from build123d import *

# Parameters (mm, degrees)
F0_R     = 40.75
F0_R_2   = 39.55
F1_DEPTH = 50
F0_R_3   = 57.8499995172
F0_R_4   = 43.75
F0_R_5   = 42.55
F2_DEPTH = 1
F3_DEPTH = 50


with BuildPart() as f1:
    # F0 (on Top) → F1 (new body)
    with BuildSketch(Plane.XY):
        Circle(F0_R)
        Circle(F0_R_2, mode=Mode.SUBTRACT)
    extrude(amount=-F1_DEPTH)

    # F0 (on Top) → F2 (join)
    with BuildSketch(Plane.XY):
        Circle(F0_R_3)
        Circle(F0_R_4, mode=Mode.SUBTRACT)
        Circle(F0_R_4)
        Circle(F0_R_5, mode=Mode.SUBTRACT)
        Circle(F0_R_5)
        Circle(F0_R, mode=Mode.SUBTRACT)
        Circle(F0_R)
        Circle(F0_R_2, mode=Mode.SUBTRACT)
    extrude(amount=F2_DEPTH)

    # F0 (on Top) → F3 (join)
    with BuildSketch(Plane.XY):
        Circle(F0_R_4)
        Circle(F0_R_5, mode=Mode.SUBTRACT)
    extrude(amount=F3_DEPTH)


solid = f1.part
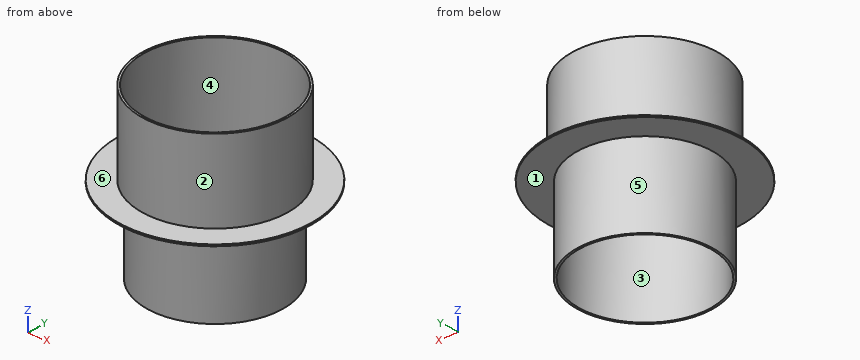
Design review of the part built by this model. Coordinates are the model's own, in mm. Face numbers are marked on the shaded views. A direction names the side the tool comes from. Give positions to 0.01 mm unless a question says otherwise; leave off trailing zeros. Order: outer loops, then holes, each group sorted by start corner. A loop starts at its lowest first (then second) coordinate and runs counter-clockwise, first axis right, second up. Notation, with made-up numbers: (33.25, 62) - (75.25, 62) arc R10 cw to (75.25, 70) - close; hole circle Ø7 at (-3.75, 69.5). An arc over 180 degrees is marked (long way). Use CSV: the item, a comma, the result in double quotes. Start each with the question number.
Q1. Draft analysis for pull direction X (two halves, no side actions). For the marked faces 1, 2, 3 and 4, state which applies: pulls with the +X half, pulls with the -X half, needs draft (parallel to the pull), parting line crosses it, or undercut.
Q2. For P1, Ø6, axis at y = -1, z = -31, coming from the +X side; P2, Ø6, axis at x = -4, z = 3.5, coming from the +Y side; P3, Ø1.5, axis at x = 38.5, y = 22, coming from the +Z side; P4, Ø2, axis at x = 39.5, y = 40, coming from the +Z side, all flat-tipped, find the tip position at first contact; note any pin that passes through.
Q3. Machinability: for the marked faces 5 and 6, which of the approach directions +Z, -Z, +X, -X, +Y, -Y give a long, thin tool a straight path to every point of the face, cutting with its end or side? Answer none if there is none.
Q4. For line 1 (X direction, y = 0, z = 16); line 2 (Y direction, x = 0, z = -37), list the stretches that pass through material, from the lowest coordinate up.
Q5. Take a section at A-A (y = 0). State the section outline as (x, z) points, and give its area (3 significant figures).
Q6. Take a section at C-C (z = -35). State the section outline as (x, y) points, and give its area (3 significant figures).
Q7. Take a section at D-D (z = 8.5). State the section outline as (x, y) points.
Calculated:
1,face 1,"needs draft"
1,face 2,"parting line crosses it"
1,face 3,"undercut"
1,face 4,"undercut"
2,P1,"stops at x = 40.75"
2,P2,"stops at y = 57.8"
2,P3,"stops at z = 50"
2,P4,"stops at z = 1"
3,face 5,"-Z"
3,face 6,"+Z"
4,line 1,"x = -43.75 to -42.55, 42.55 to 43.75"
4,line 2,"y = -40.75 to -39.55, 39.55 to 40.75"
5,outline,"(-57.85, 0) - (-40.75, 0) - (-40.75, -50) - (-39.55, -50) - (-39.55, 1) - (-42.55, 1) - (-42.55, 50) - (-43.75, 50) - (-43.75, 1) - (-57.85, 1) - close; (39.55, -50) - (40.75, -50) - (40.75, 0) - (57.85, 0) - (57.85, 1) - (43.75, 1) - (43.75, 50) - (42.55, 50) - (42.55, 1) - (39.55, 1) - close"
5,area,"274 mm²"
6,outline,"circle Ø81.5 at (0, 0); hole circle Ø79.1 at (0, 0)"
6,area,"303 mm²"
7,outline,"circle Ø87.5 at (0, 0); hole circle Ø85.1 at (0, 0)"
